Can you work these out from the model? Positions are in its coordinate system, mm. A direction names the side the tool comes from. Give positions to 0.01 mm unless a question says otherwise; leave off trailing zeros. Order: outer loops, then holes, each group sorted by start corner. A loop starts at its lowest first (then second) coordinate and runs counter-clockwise, first axis right, second up. Notation, with made-up numbers: M -11.75,42.5 L 41.25,42.5 A13 ccw 41.25,49.5 Z; hole C 17,82.5 d8. An arc over 180 degrees is marked long. Use one line per item in the form item = value. Start each with the question number.
1. I need wall thicknesses on L1, parallel to X at y = 25.65, z = 13; L2, parallel to X at y = 2.7, z = -36.65; L3, parallel to Y at x = 21, z = 8.5. Which ranges of each line are inside material? Lowest first, please.
2. I want a section at B-B, the plane x = 21.15. List the corners of the cut face in (y, z) for me, and give its area (3 significant figures).
3. We'd pull the mould along X, two halves only. Please class faces 1 (the face through (-3, -11, -10)), 2 (the face through (10, 3, -16)), 3 (the face through (5.771, 2.754, -39.397)): +X half, -X half, draft (parallel to the pull), parting line (faces both ways), or undercut.
4. Will these pins go through, and if not, where does the flat tip stop? P1, Ø6.5, axis at x = 10, y = 13, coming from the -Z side; P2, Ø6.5, axis at x = 10, z = 13, coming from the -Y side; P3, Ø4.5, axis at x = 6.5, z = -6.5, coming from the +Y side; P4, Ø6, axis at x = 5, z = 4.5, coming from the -Y side.
5. I want a section at D-D, the plane z = -36.65. List the corners of the cut face in (x, y) for me.
6. I want a section at C-C, the plane z = -21.15. List the corners of the cut face in (x, y) for me, and give its area (3 significant figures).
7. For faces 4 (the face through (21, -21, 3)), 5 (the face through (21, -20, 0)), 6 (the face through (7.509, 2.754, -7.677)), which set-ups out of +Z, -Z, +X, -X, +Y, -Y let a thin tool reach every point of the face, with its end or its side?
8. I want a section at A-A, the plane y = 13. List the corners of the cut face in (x, z) for me, and give its area (3 significant figures).
```python
from build123d import *

# Parameters (mm, degrees)
SKETCH1_W                = 42.3
SKETCH1_H                = 42.3
SKETCH1_R                = 11.5
BOSS_EXTRUDE2_DEPTH      = 3
SKETCH2_R                = 1.5
CUT_EXTRUDE1_DEPTH       = 3
BOSS_EXTRUDE3_DEPTH      = 3
BOSS_EXTRUDE3_DEPTH_BACK = 42
SKETCH3_W                = 3
SKETCH3_H                = 42.3
SKETCH5_W                = 45.3
SKETCH5_H                = 45
BOSS_EXTRUDE4_DEPTH      = 3
CUT_EXTRUDE3_DEPTH       = 74.092954517
CUT_EXTRUDE3_DEPTH_BACK  = 3
SKETCH8_W                = 45.3
SKETCH8_H                = 45
BOSS_EXTRUDE5_DEPTH      = 3
SKETCH12_W               = 48.3
SKETCH12_H               = 3
BOSS_EXTRUDE6_DEPTH      = 23
SKETCH14_W               = 48.3
SKETCH14_H               = 3
BOSS_EXTRUDE7_DEPTH      = 20
SKETCH17_R               = 2.75
CUT_EXTRUDE5_DEPTH       = 0.5
CUT_EXTRUDE6_DEPTH       = 75.869085743
CUT_EXTRUDE6_DEPTH_BACK  = 3
SKETCH19_W               = 48.3
SKETCH19_H               = 3
BOSS_EXTRUDE8_DEPTH      = 20
SKETCH21_R               = 1.5
CUT_EXTRUDE7_DEPTH       = 20
SKETCH23_R               = 2.75
CUT_EXTRUDE9_DEPTH       = 1
SKETCH26_R               = 2.75
CUT_EXTRUDE10_DEPTH      = 1
SKETCH27_R               = 1.3
SKETCH27_R_2             = 1.5
CUT_EXTRUDE11_DEPTH      = 41
SKETCH30_R               = 2.75
CUT_EXTRUDE12_DEPTH      = 1
SKETCH31_R               = 2.75
CUT_EXTRUDE13_DEPTH      = 1
CUT_EXTRUDE14_START      = -1
SKETCH32_R               = 2.75
CUT_EXTRUDE14_DEPTH      = 1
CUT_EXTRUDE15_START      = -1
SKETCH33_R               = 2.75
CUT_EXTRUDE15_DEPTH      = 1
SKETCH38_W               = 42.3
SKETCH38_H               = 42.3
CUT_EXTRUDE16_DEPTH      = 1


with BuildPart() as part:
    # Sketch1 → Boss-Extrude2 (new body)
    with BuildSketch(Plane(origin=(0, 0, 0), x_dir=(1, 0, 0), z_dir=(0, 1, 0))):
        with Locations((21.15, 21.15)):
            Rectangle(SKETCH1_W, SKETCH1_H)
        with Locations(Location((21.15, 21.15, 0), (0, 0, 270))):
            Circle(SKETCH1_R, mode=Mode.SUBTRACT)
    extrude(amount=BOSS_EXTRUDE2_DEPTH)

    # Sketch2 → Cut-Extrude1 (cut)
    with BuildSketch(Plane(origin=(0, 3, 0), x_dir=(1, 0, 0), z_dir=(0, 1, 0))):
        with Locations(Location((5.65, 5.65, 0), (0, 0, 270))):
            Circle(SKETCH2_R)
        with Locations(Location((5.65, 36.65, 0), (0, 0, 270))):
            Circle(SKETCH2_R)
        with Locations(Location((36.65, 36.65, 0), (0, 0, 270))):
            Circle(SKETCH2_R)
        with Locations(Location((36.65, 5.65, 0), (0, 0, 270))):
            Circle(SKETCH2_R)
    extrude(amount=-CUT_EXTRUDE1_DEPTH, mode=Mode.SUBTRACT)

    # Sketch3 → Boss-Extrude3 (add, two sides: drawn at the far end of the back side and taken through both)
    with BuildSketch(Plane(origin=(0, 0, 0), x_dir=(1, 0, 0), z_dir=(0, 1, 0)).offset(-BOSS_EXTRUDE3_DEPTH_BACK)):
        with Locations((-1.5, 21.15)):
            Rectangle(SKETCH3_W, SKETCH3_H)
    extrude(amount=BOSS_EXTRUDE3_DEPTH + BOSS_EXTRUDE3_DEPTH_BACK)

    # Sketch5 → Boss-Extrude4 (add)
    with BuildSketch(Plane.XY):
        with Locations((19.65, -19.5)):
            Rectangle(SKETCH5_W, SKETCH5_H)
    extrude(amount=BOSS_EXTRUDE4_DEPTH)

    # Sketch6 → Cut-Extrude3 (cut, two sides: drawn at the far end of the back side and taken through both)
    with BuildSketch(Plane(origin=(0, 0, 0), x_dir=(0, 0, -1), z_dir=(1, 0, 0)).offset(-CUT_EXTRUDE3_DEPTH_BACK)):
        Polygon((-94.768878565, -136.096758859), (0, -42), (42.3, 0), (137.068878565, 94.096758859), (325.262396283, -95.440998271), (93.424639153, -325.634515989), align=None)
    extrude(amount=CUT_EXTRUDE3_DEPTH + CUT_EXTRUDE3_DEPTH_BACK, mode=Mode.SUBTRACT)

    # Sketch8 → Boss-Extrude5 (add)
    with BuildSketch(Plane(origin=(42.3, 0, 0), x_dir=(0, 0, -1), z_dir=(1, 0, 0))):
        with Locations((19.65, -19.5)):
            Rectangle(SKETCH8_W, SKETCH8_H)
    extrude(amount=BOSS_EXTRUDE5_DEPTH)

    # Sketch12 → Boss-Extrude6 (add)
    with BuildSketch(Plane(origin=(0, 3, 0), x_dir=(1, 0, 0), z_dir=(0, 1, 0))):
        with Locations((21.15, -1.5)):
            Rectangle(SKETCH12_W, SKETCH12_H)
    extrude(amount=BOSS_EXTRUDE6_DEPTH)

    # Sketch14 → Boss-Extrude7 (add)
    with BuildSketch(Plane.XY.offset(3)):
        with Locations((21.15, 24.5)):
            Rectangle(SKETCH14_W, SKETCH14_H)
    extrude(amount=BOSS_EXTRUDE7_DEPTH)

    # Sketch17 → Cut-Extrude5 (cut)
    with BuildSketch(Plane(origin=(0, 3, 0), x_dir=(1, 0, 0), z_dir=(0, 1, 0))):
        with Locations(Location((36.65, 36.65, 0), (0, 0, 270))):
            Circle(SKETCH17_R)
        with Locations(Location((36.65, 5.65, 0), (0, 0, 270))):
            Circle(SKETCH17_R)
        with Locations(Location((5.65, 36.65, 0), (0, 0, 270))):
            Circle(SKETCH17_R)
        with Locations(Location((5.65, 5.65, 0), (0, 0, 270))):
            Circle(SKETCH17_R)
    extrude(amount=-CUT_EXTRUDE5_DEPTH, mode=Mode.SUBTRACT)

    # Sketch18 → Cut-Extrude6 (cut, two sides: drawn at the far end of the back side and taken through both)
    with BuildSketch(Plane.ZY.offset(-42.3).offset(-CUT_EXTRUDE6_DEPTH_BACK)):
        Polygon((-163.053000202, 119.896595945), (-42.3, 0), (0, -42), (120.753000202, -161.896595945), (-119.040191688, -403.402596349), (-402.846192092, -121.609404459), align=None)
    extrude(amount=CUT_EXTRUDE6_DEPTH + CUT_EXTRUDE6_DEPTH_BACK, mode=Mode.SUBTRACT)

    # Sketch19 → Boss-Extrude8 (add)
    with BuildSketch(Plane.XY.offset(3)):
        with Locations((21.15, 1.5)):
            Rectangle(SKETCH19_W, SKETCH19_H)
    extrude(amount=BOSS_EXTRUDE8_DEPTH)

    # Sketch21 → Cut-Extrude7 (cut)
    with BuildSketch(Plane(origin=(0, 0, 0), x_dir=(-1, 0, 0), z_dir=(0, 0, -1))):
        with Locations((-32.301370807, 13)):
            Circle(SKETCH21_R)
        with Locations((-10, 13)):
            Circle(SKETCH21_R)
    extrude(amount=-CUT_EXTRUDE7_DEPTH, mode=Mode.SUBTRACT)

    # Sketch23 → Cut-Extrude9 (cut)
    with BuildSketch(Plane(origin=(0, 0, 0), x_dir=(-1, 0, 0), z_dir=(0, 0, -1))):
        with Locations((-10, 13)):
            Circle(SKETCH23_R)
    extrude(amount=-CUT_EXTRUDE9_DEPTH, mode=Mode.SUBTRACT)

    # Sketch26 → Cut-Extrude10 (cut)
    with BuildSketch(Plane(origin=(0, 0, 0), x_dir=(-1, 0, 0), z_dir=(0, 0, -1))):
        with Locations((-32.3, 13)):
            Circle(SKETCH26_R)
    extrude(amount=-CUT_EXTRUDE10_DEPTH, mode=Mode.SUBTRACT)

    # Sketch27 → Cut-Extrude11 (cut)
    with BuildSketch(Plane(origin=(0, 26, 0), x_dir=(1, 0, 0), z_dir=(0, 1, 0))):
        with Locations(Location((10, -13, 0), (0, 0, 270))):
            Circle(SKETCH27_R)
        with Locations(Location((32.3, -13, 0), (0, 0, 270))):
            Circle(SKETCH27_R_2)
    extrude(amount=-CUT_EXTRUDE11_DEPTH, mode=Mode.SUBTRACT)

    # Sketch30 → Cut-Extrude12 (cut)
    with BuildSketch(Plane(origin=(0, 26, 0), x_dir=(1, 0, 0), z_dir=(0, 1, 0))):
        with Locations(Location((10, -13, 0), (0, 0, 270))):
            Circle(SKETCH30_R)
    extrude(amount=-CUT_EXTRUDE12_DEPTH, mode=Mode.SUBTRACT)

    # Sketch31 → Cut-Extrude13 (cut)
    with BuildSketch(Plane(origin=(0, 26, 0), x_dir=(1, 0, 0), z_dir=(0, 1, 0))):
        with Locations(Location((32.3, -13, 0), (0, 0, 270))):
            Circle(SKETCH31_R)
    extrude(amount=-CUT_EXTRUDE13_DEPTH, mode=Mode.SUBTRACT)

    # Sketch32 → Cut-Extrude14 (cut)
    with BuildSketch(Plane.XZ.offset(CUT_EXTRUDE14_START)):
        with Locations(Location((32.3, 13, 0), (0, 0, 90))):
            Circle(SKETCH32_R)
    extrude(amount=CUT_EXTRUDE14_DEPTH, mode=Mode.SUBTRACT)

    # Sketch33 → Cut-Extrude15 (cut)
    with BuildSketch(Plane.XZ.offset(CUT_EXTRUDE15_START)):
        with Locations(Location((10, 13, 0), (0, 0, 90))):
            Circle(SKETCH33_R)
    extrude(amount=CUT_EXTRUDE15_DEPTH, mode=Mode.SUBTRACT)

    # Sketch38 → Cut-Extrude16 (cut)
    with BuildSketch(Plane(origin=(0, 0, 0), x_dir=(-1, 0, 0), z_dir=(0, -1, 0))):
        with Locations((-21.15, 21.15)):
            Rectangle(SKETCH38_W, SKETCH38_H)
    extrude(amount=-CUT_EXTRUDE16_DEPTH, mode=Mode.SUBTRACT)


solid = part.part
```
Check result:
q1.L1 = -3 to 7.25, 12.75 to 29.55, 35.05 to 45.3
q1.L2 = -3 to 2.9, 8.4 to 33.9, 39.4 to 45.3
q1.L3 = 0 to 3, 23 to 26
q2.outline = M -42,0 L 1,0 L 1,-9.65 L 3,-9.65 L 3,0 L 26,0 L 26,23 L 23,23 L 23,3 L 3,3 L 3,23 L 0,23 L 0,3 L -42,3 Z; M 1,-42.3 L 3,-42.3 L 3,-32.65 L 1,-32.65 Z
q2.area = 363 mm2
q3.face_1 = -X half
q3.face_2 = draft
q3.face_3 = undercut
q4.P1 = 0
q4.P2 = 0
q4.P3 = 3
q4.P4 = -42
q5.outline = M -3,-5.61 L 0,-5.61 L 0,1 L 4.15,1 L 4.15,2.5 L 2.9,2.5 L 2.9,3 L -3,3 Z; M 7.15,1 L 35.15,1 L 35.15,2.5 L 33.9,2.5 L 33.9,3 L 8.4,3 L 8.4,2.5 L 7.15,2.5 Z; M 38.15,1 L 42.3,1 L 42.3,-5.61 L 45.3,-5.61 L 45.3,3 L 39.4,3 L 39.4,2.5 L 38.15,2.5 Z
q6.outline = M -3,-21 L 0,-21 L 0,1 L 9.65,1 L 9.65,3 L -3,3 Z; M 32.65,1 L 42.3,1 L 42.3,-21 L 45.3,-21 L 45.3,3 L 32.65,3 Z
q6.area = 183 mm2
q7.face_4 = +Z, +X, -X, -Y
q7.face_5 = -Z, -Y
q7.face_6 = +Y
q8.outline = M -3,0 L 7.25,0 L 7.25,1 L 8.5,1 L 8.5,3 L -3,3 Z; M 11.5,1 L 12.75,1 L 12.75,0 L 29.55,0 L 29.55,1 L 30.8,1 L 30.8,3 L 11.5,3 Z; M 33.8,1 L 35.05,1 L 35.05,0 L 45.3,0 L 45.3,3 L 33.8,3 Z
q8.area = 122 mm2
